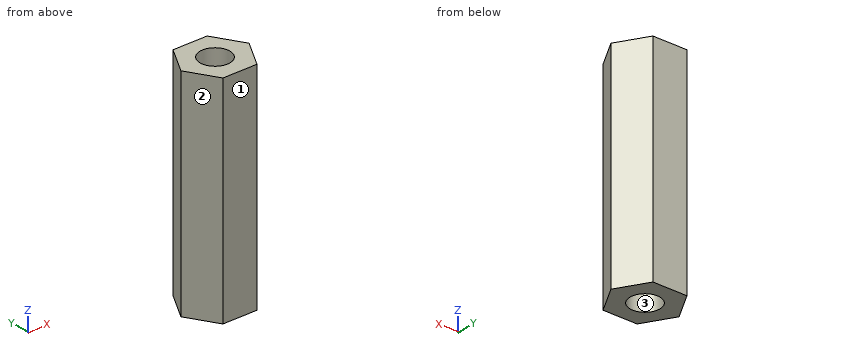
Autodesk Inventor part; units mm, degrees
ref_plane "YZ Plane" through (0, 0, 0) normal (1, 0, 0) x (0, 1, 0)
ref_plane "XZ Plane" through (0, 0, 0) normal (0, 1, 0) x (-1, 0, 0)
ref_plane "XY Plane" through (0, 0, 0) normal (0, 0, 1) x (1, 0, 0)
sketch "Sketch1" plane through (0, 0, 0) normal (0, 0, 1) x (1, 0, 0)
  line L0 (7.9674, 0) -> (3.9837, -6.9)
  line L1 (3.9837, -6.9) -> (-3.9837, -6.9)
  line L2 (-3.9837, -6.9) -> (-7.9674, 0)
  line L3 (-7.9674, 0) -> (-3.9837, 6.9)
  line L4 (-3.9837, 6.9) -> (3.9837, 6.9)
  line L5 (3.9837, 6.9) -> (7.9674, 0)
  line L6 (3.4641, 0) -> (1.7321, -3)
  line L7 (1.7321, -3) -> (-1.7321, -3)
  line L8 (-1.7321, -3) -> (-3.4641, 0)
  line L9 (-3.4641, 0) -> (-1.7321, 3)
  line L10 (-1.7321, 3) -> (1.7321, 3)
  line L11 (1.7321, 3) -> (3.4641, 0)
  point P0 (0, 0)
  point P1 (0, 0)
  point P2 (0, 0)
  dimension "d0" = 13.8
  dimension "d1" = 6
extrude "Extrusion1" add sketch "Sketch1" along normal blind 50
sketch "Sketch2" plane through (0, 0, 50) normal (0, 0, 1) x (1, 0, 0)
  line L0 (1.7321, -3) -> (-1.7321, -3)
  circle A0 centre (0, 0) radius 3.4641
extrude "Extrusion2" cut sketch "Sketch2" against normal blind 50
properties part number "Montaje Manguera"
Design review of the part built by this model. Coordinates are the model's own, in mm. Face numbers are marked on the shaded views. Round coordinates to 2 decimals unless told otherwise and drop trailing zeros. Order: outer loops, then holes, each group sorted by start corner. A loop starts at its lowest first (then second) coordinate and runs counter-clockwise, first axis right, second up. Notation, with made-up numbers: (11.5, 37.5) - (62.5, 37.5) arc R23 cw to (62.5, 58.5) - close; hole circle Ø3 at (42, 60). An arc over 180 degrees is marked (long way). One line per question, with ' | ' between items.
Item 1: Take a section at B-B, the plane z = 6. Write out the cut boundary in (x, y).
Checks:
outline: (-7.97, 0) - (-3.98, -6.9) - (3.98, -6.9) - (7.97, 0) - (3.98, 6.9) - (-3.98, 6.9) - close; hole circle Ø6.93 at (0, 0)
Item 2: Take a section at C-C, the plane y = 0.5. Write out the cut boundary in (x, z), then the cut area to 3 significant figures.
Checks:
outline: (-7.68, 0) - (-3.43, 0) - (-3.43, 50) - (-7.68, 50) - close; (3.43, 0) - (7.68, 0) - (7.68, 50) - (3.43, 50) - close | area: 425 mm²
Item 3: Take a section at A-A, the plane x = 0. Write out the cut boundary in (y, z).
Checks:
outline: (-6.9, 0) - (-3.46, 0) - (-3.46, 50) - (-6.9, 50) - close; (3.46, 0) - (6.9, 0) - (6.9, 50) - (3.46, 50) - close
Item 4: Take a section at D-D, the plane y = -5.25. Write out the cut boundary in (x, z).
Checks:
outline: (-4.94, 0) - (4.94, 0) - (4.94, 50) - (-4.94, 50) - close
Item 5: Draft analysis for pull direction X (two halves, no side actions). For the marked faces 1, 2 and 3, state which applies: +X half, -X half, draft (parallel to the pull), parting line (faces both ways), or undercut.
Checks:
face 1: draft | face 2: -X half | face 3: undercut
Item 6: For P1, Ø1, axis at y = 1.5, z = 34, coming from the -X side; P2, Ø1, axis at x = -5, z = 37.5, coming from the -Y side; P3, Ø1, axis at y = 2.5, z = 6, coming from the -X side, all flat-tipped, find the tip position at first contact; note any pin that passes through.
Checks:
P1: x = -7.39 | P2: y = -6.01 | P3: x = -6.81
Item 7: Wall thickness on line 1 (X direction, y = 0, z = 39); line 2 (Y direction, x = 0, z = 23.5); line 3 (X direction, y = -2.5, z = 35): over which ranges is each line inside the solid? List them lowest first. Write a range as [from, to].
Checks:
line 1: [-7.97, -3.46], [3.46, 7.97] | line 2: [-6.9, -3.46], [3.46, 6.9] | line 3: [-6.52, -2.4], [2.4, 6.52]
